For this review, take the finished solid that the model builds, in its own axes (mm). A direction names the side the tool comes from. Round coordinates to 2 decimals unless told otherwise and drop trailing zeros. Order: outer loops, then holes, each group sorted by start corner. A loop starts at its lowest first (then second) coordinate and runs counter-clockwise, first axis right, second up. Notation, with made-up numbers: (43.25, 48.5) -> (88.25, 48.5) arc R19 ccw to (88.25, 71.5) -> close; hole circle Ø9 at (-23.5, 13). An arc over 180 degrees is marked (long way). Put each result on its own line as item: value. Start each with the question number.
```python
from build123d import *

# Parameters (mm, degrees)
SKETCH_1_W          = 5
SKETCH_1_H          = 5
EXTRUDE_1_DEPTH     = 8
SKETCH_2_W          = 7
SKETCH_2_H          = 7
EXTRUDE_2_DEPTH     = 2
SKETCH_3_R          = 1.5
CUT_EXTRUDE_1_DEPTH = 5


with BuildPart() as part:
    # 草图1 → 凸台-拉伸1 (new body)
    with BuildSketch(Plane.XY):
        Rectangle(SKETCH_1_W, SKETCH_1_H)
    extrude(amount=EXTRUDE_1_DEPTH)

    # 草图2 → 凸台-拉伸2 (add)
    with BuildSketch(Plane(origin=(0, 0, 0), x_dir=(-1, 0, 0), z_dir=(0, 0, -1))):
        Rectangle(SKETCH_2_W, SKETCH_2_H)
    extrude(amount=-EXTRUDE_2_DEPTH)

    # 草图3 → 切除-拉伸1 (cut)
    with BuildSketch(Plane(origin=(0, 0, 0), x_dir=(-1, 0, 0), z_dir=(0, 0, -1))):
        Circle(SKETCH_3_R)
    extrude(amount=-CUT_EXTRUDE_1_DEPTH, mode=Mode.SUBTRACT)


solid = part.part
```
Item 1: Tool access review of faces 5 (the face through (0, 2.5, 5)), 6 (the face through (1.5, 0.07, 2.46)), 7 (the face through (-2.5, 0, 5)): name each direction out of +Z, -Z, +X, -X, +Y, -Y from which nothing blocks a thin tool from reaching the whole face with its end or side.
Item 2: Insertion check: pin 1 Ø1.5 at (y, z) = (1, 6) entering from -X; pin 2 Ø2.5 at (x, y) = (0, 0) entering from -Z; pin 3 Ø4 at (x, z) = (-2, 6.5) entering from +Y. Each pin has a flat end and moves straight along its axis. Give the tip position at first contact, or say it passes through.
Item 3: Mouldability with a two-part tool opening along Y and no side actions: class faces 1 (the face through (0, 3.5, 1)), 2 (the face through (0, 0, 5)), 3 (the face through (0, -2.5, 5)), 4 (the face through (2.5, 0, 5)) as +Y half, -Y half, draft (parallel to the pull), parting line (faces both ways), or undercut.
Item 4: Consider section D-D, the plane y = 0. Write out the cut boundary in (x, z), plus the area to 3 significant figures.
Item 5: For L1, parallel to Y at x = 0, z = 3.5; L2, parallel to Z at x = -1.5, y = -3; L3, parallel to X at y = 1.25, z = 5.75, list the stretches that pass through material, from the lowest coordinate up.
Item 6: Consider section A-A, the plane x = 2. Write out the cut boundary in (y, z).
Item 7: Consider section C-C, the plane z = 4.5. Write out the cut boundary in (x, y).
Evaluation:
1. face 5: +Z, +X, -X, +Y
1. face 6: -Z
1. face 7: +Z, -X, +Y, -Y
2. pin 1: stops at x = -2.5
2. pin 2: stops at z = 5
2. pin 3: stops at y = 2.5
3. face 1: +Y half
3. face 2: undercut
3. face 3: -Y half
3. face 4: draft
4. outline: (-3.5, 0) -> (-1.5, 0) -> (-1.5, 5) -> (1.5, 5) -> (1.5, 0) -> (3.5, 0) -> (3.5, 2) -> (2.5, 2) -> (2.5, 8) -> (-2.5, 8) -> (-2.5, 2) -> (-3.5, 2) -> close
4. area: 29.0 mm^2
5. L1: y = -2.5 to -1.5, 1.5 to 2.5
5. L2: z = 0 to 2
5. L3: x = -2.5 to 2.5
6. outline: (-3.5, 0) -> (3.5, 0) -> (3.5, 2) -> (2.5, 2) -> (2.5, 8) -> (-2.5, 8) -> (-2.5, 2) -> (-3.5, 2) -> close
7. outline: (-2.5, -2.5) -> (2.5, -2.5) -> (2.5, 2.5) -> (-2.5, 2.5) -> close; hole circle Ø3 at (0, 0)
